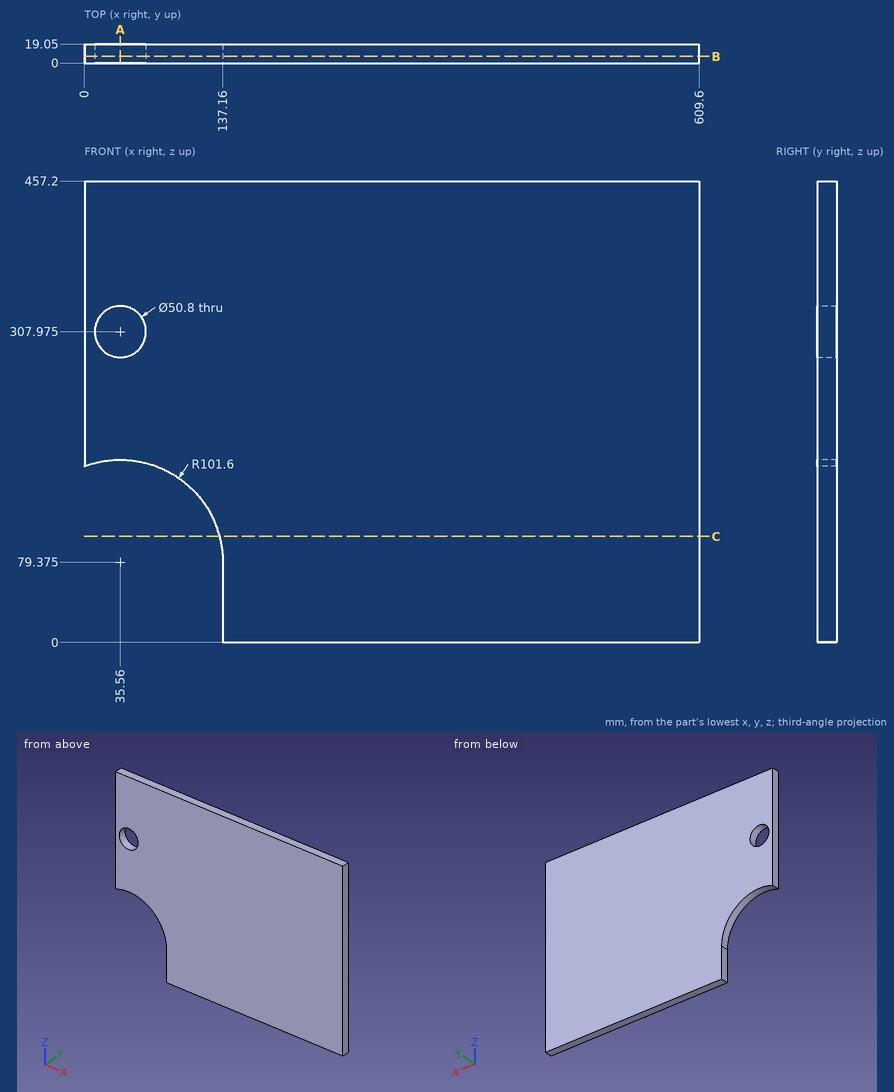
Check sheet for the drawn part. Datum: minimum x, y, z corner. Units: mm. Give positions to 0.01 mm unless a question says otherwise; leave off trailing zeros. Loops run counter-clockwise (first coordinate to the right, second up) from the corner with the lowest first, then second, coordinate; pieces in that order, holes last.
1) Thickness scan on line 1 along X through (y, z) = (17.25, 308); line 2 along X through (y, z) = (5.25, 30); line 3 along X through (y, z) = (16.5, 304). Record the ranges inside material, lowest first.
2) Depth check by flat-ended pin: pin 1 Ø5.5 at (y, z) = (5.5, 32) entering from -X; pin 2 Ø3 at (x, z) = (210.5, 266.5) entering from -Y; pin 3 Ø1 at (x, y) = (122.5, 15.5) entering from -Z; pin 4 Ø6 at (y, z) = (10.5, 145.5) entering from -X. Enter the tip coordinate at first touch or a pass-through.
3) Sectioned sample at C-C, the plane z = 105. Enter the section's corners in (x, y).
4) Sectioned sample at A-A, the plane x = 35.56. Enter the section's corners in (y, z) (3 decimals).
5) Sectioned sample at B-B, the plane y = 6.75. Enter the section's corners in (x, z) (3 decimals), then the cut area to 3 significant figures.
Answers:
1. line 1: x = 0 to 10.16, 60.96 to 609.6
1. line 2: x = 137.16 to 609.6
1. line 3: x = 0 to 10.47, 60.65 to 609.6
2. pin 1: stops at x = 137.16
2. pin 2: stops at y = 0
2. pin 3: stops at z = 131.11
2. pin 4: stops at x = 110.02
3. outline: (133.88, 0) - (609.6, 0) - (609.6, 19.05) - (133.88, 19.05) - close
4. outline: (0, 180.975) - (19.05, 180.975) - (19.05, 282.575) - (0, 282.575) - close; (0, 333.375) - (19.05, 333.375) - (19.05, 457.2) - (0, 457.2) - close
5. outline: (0, 174.549) arc R101.6 cw to (137.16, 79.375) - (137.16, 0) - (609.6, 0) - (609.6, 457.2) - (0, 457.2) - close; hole circle Ø50.8 at (35.56, 307.975)
5. area: 254,000 mm2
